The model under review builds one solid part; all positions refer to its coordinate system, in mm. Face numbers are marked on the shaded views. Coordinates: 2 decimals unless noted, no trailing zeros. Write each loop counter-clockwise with the first axis right and the second up, starting at its lowest first coordinate (ties: lowest second). Pieces come first, ordered by that corner, then holes. Notation, with made-up numbers: (29.5, -31) - (63.5, -31) arc R11 ccw to (63.5, -22) - close; hole circle Ø3 at (-25.75, 33). An arc over 180 degrees is marked (long way). Use one line per item in the form item = value. Start each with the question number.
Autodesk Inventor part; units mm, degrees
ref_plane "YZ Plane" through (0, 0, 0) normal (1, 0, 0) x (0, 1, 0)
ref_plane "XZ Plane" through (0, 0, 0) normal (0, 1, 0) x (-1, 0, 0)
ref_plane "XY Plane" through (0, 0, 0) normal (0, 0, 1) x (1, 0, 0)
sketch "Sketch1" plane through (0, 0, 0) normal (0, 1, 0) x (-1, 0, 0)
  line L0 (0, 13.9753) -> (0, -99.2247)
  line L1 (0, -99.2247) -> (60, -99.2247)
  line L2 (0, 13.9753) -> (23, -3.0438)
  line L3 (23, -3.0438) -> (60, -3.0438)
  line L4 (60, -3.0438) -> (60, -99.2247)
  point P0 (0, 0)
  dimension "d0" = 113.2
  dimension "d2" = 60
  dimension "d5" = 53.5
  dimension "d6" = 37
extrude "Extrusion1" add sketch "Sketch1" along normal blind 2
sketch "Sketch2" plane through (-60, 0, -3.0438) normal (0, 0, 1) x (1, 0, 0)
  line L0 (0, 0) -> (0, 2)
  line L1 (60, 0) -> (0, 0)
  line L2 (0, 2) -> (37, 2)
  line L3 (37, 2) -> (37, 0)
  line L4 (37, 0) -> (0, 0)
  line L5 (0, 0) -> (0, 2)
  line L6 (37, 0) -> (37, 2)
  point P0 (37, 1)
extrude "Extrusion2" add sketch "Sketch2" along normal blind 0.1
properties part number "tapa4_3DPrint"
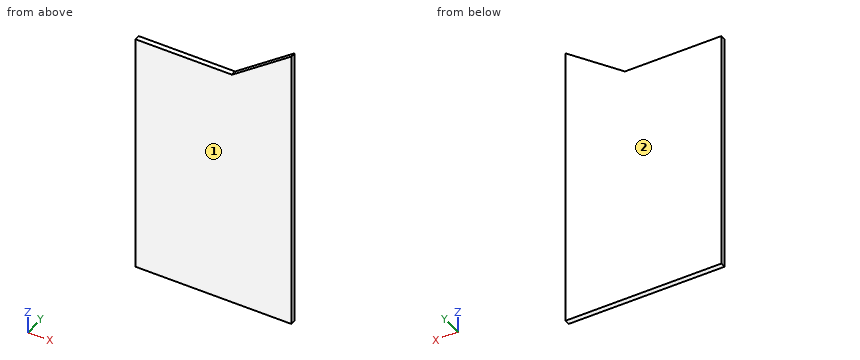
1. For L1, parallel to Z at x = -30, y = 0.5; L2, parallel to Z at x = -21, y = 1.95; L3, parallel to X at y = 1.05, z = 7, list the stretches that pass through material, from the lowest coordinate up.
2. Take a section at B-B (x = -53). State the section outline as (y, z) points.
3. Take a section at C-C (z = 1). State the section outline as (x, y) points, plus the area to 3 significant figures.
4. The part is to be moulded in two halves that separate along Y. For the marked faces 1 and 2, say which applies: released by +Y, released by -Y, zero draft, split by the parting line, or undercut.
5. For P1, Ø1, axis at x = -49.5, y = 1, coming from the +Z side, flat-tipped, find the tip position at first contact; note if it passes through.
6. Take a section at A-A (y = 0.6). State the section outline as (x, z) points, plus the area to 3 significant figures.
Returned:
q1.L1 = -99.22 to -2.94
q1.L2 = -99.22 to -1.56
q1.L3 = -9.43 to 0
q2.outline = (0, -99.22) - (2, -99.22) - (2, -2.94) - (0, -2.94) - close
q3.outline = (-17.54, 0) - (0, 0) - (0, 2) - (-17.54, 2) - close
q3.area = 35.1 mm²
q4.face_1 = released by -Y
q4.face_2 = released by +Y
q5.P1 = -2.94
q6.outline = (-60, -99.22) - (0, -99.22) - (0, 13.98) - (-23, -3.04) - (-23, -2.94) - (-60, -2.94) - close
q6.area = 5,970 mm²
